Input: part model. Units: mm. Frame: model coordinates. A direction names the side the tool comes from. Round coordinates to 2 decimals unless told otherwise and drop trailing zeros. Write each loop counter-clockwise with the first axis right and the second up, starting at its lowest first coordinate (ties: lowest second). Pieces come first, ordered by that corner, then holes. Notation, with made-up numbers: (62, 26.25) -> (95, 26.25) arc R7 cw to (95, 35.25) -> close; hole circle Ø1 at (36, 61). An arc over 180 degrees is marked (long way). Use CSV: the item, a comma, the result in double quotes.
Autodesk Inventor part; units mm, degrees
ref_plane "Arbeitsebene1" through (-276.74, -145.36, 4.8625) normal (0, 0, 1) x (1, 0, 0)
ref_plane "YZ Plane" through (0, 0, 0) normal (1, 0, 0) x (0, 1, 0)
ref_plane "XZ Plane" through (0, 0, 0) normal (0, 1, 0) x (-1, 0, 0)
sketch "Skizze1" plane through (0, 0, 0) normal (0, 0, 1) x (1, 0, 0)
  circle A0 centre (-271.1, -102.4) radius 2.25
  circle A1 centre (-271, -139.7) radius 2.25
  circle A2 centre (-140.5, -84.3) radius 2.25
  circle A3 centre (-161.5, -132.1) radius 2.25
  circle A4 centre (-28.4, -139.7) radius 2.25
  circle A5 centre (-28.2, -86.4) radius 2.25
  circle A6 centre (-216.6, -72.6) radius 2.25
  point P0 (0, 0)
extrude "Extrusion1" add sketch "Skizze1" along normal blind 3 contours A0 | A1 | A2 | A3 | A4 | A5
sketch "Skizze2" plane through (-216.6, -72.6, 3) normal (0, 0, 1) x (1, 0, 0)
  line L0 (-57.14, 7.74) -> (190.86, 7.74)
  arc A0 (192.36, 6.24) -> (190.86, 7.74) centre (190.86, 6.24) ccw
  line L1 (192.36, 6.24) -> (192.36, -69.76)
  arc A1 (190.86, -71.26) -> (192.36, -69.76) centre (190.86, -69.76) ccw
  line L2 (190.86, -71.26) -> (-57.14, -71.26)
  arc A2 (-58.64, -69.76) -> (-57.14, -71.26) centre (-57.14, -69.76) ccw
  line L3 (-58.64, -69.76) -> (-58.64, 6.24)
  arc A3 (-57.14, 7.74) -> (-58.64, 6.24) centre (-57.14, 6.24) ccw
  point P0 (216.6, 72.6)
ref_plane "Arbeitsebene1" through (-276.74, -145.36, 4.8625) normal (0, 0, 1) x (1, 0, 0)
extrude "Extrusion2" add sketch "Skizze2" along normal up to surface (1.8625 mm away)
sketch "Skizze3" plane through (-273.74, -143.86, 4.8625) normal (0, 0, 1) x (1, 0, 0)
  line L0 (248, 80.5) -> (0, 80.5)
  arc A0 (0, 80.5) -> (-3, 77.5) centre (0, 77.5) ccw
  line L1 (-3, 77.5) -> (-3, 1.5)
  arc A1 (-3, 1.5) -> (0, -1.5) centre (0, 1.5) ccw
  line L2 (0, -1.5) -> (248, -1.5)
  arc A2 (248, -1.5) -> (251, 1.5) centre (248, 1.5) ccw
  line L3 (251, 1.5) -> (251, 77.5)
  arc A3 (251, 77.5) -> (248, 80.5) centre (248, 77.5) ccw
  point P0 (273.74, 143.86)
extrude "Extrusion3" add sketch "Skizze3" along normal blind 5
sketch "Skizze4" plane through (-273.74, -143.86, 9.8625) normal (0, 0, 1) x (1, 0, 0)
  circle A0 centre (245.54, 57.46) radius 2.25 construction
  circle A1 centre (245.34, 4.16) radius 2.25 construction
  circle A2 centre (133.24, 59.56) radius 1.2295
  circle A3 centre (133.24, 59.56) radius 1.2295
  circle A4 centre (112.24, 11.76) radius 1.6
  circle A5 centre (57.14, 71.26) radius 2.25
  circle A6 centre (2.64, 41.46) radius 1.2295
  circle A7 centre (2.74, 4.16) radius 1.2295
  circle A8 centre (2.64, 41.46) radius 2.85
  circle A9 centre (2.74, 4.16) radius 2.85
  circle A10 centre (57.14, 71.26) radius 2.85
  circle A11 centre (112.24, 11.76) radius 2.25
  circle A12 centre (112.24, 11.76) radius 2.85
  circle A13 centre (133.24, 59.56) radius 2.25
  circle A14 centre (133.24, 59.56) radius 2.85
  circle A15 centre (245.54, 57.46) radius 2.85
  circle A16 centre (245.34, 4.16) radius 2.85
  point P0 (273.74, 143.86)
  dimension "d6" = 5.7
  dimension "d7" = 5.7
  dimension "d8" = 5.7
  dimension "d9" = 5.7
  dimension "d10" = 5.7
  dimension "d11" = 5.7
  dimension "d12" = 5.7
extrude "Extrusion4" cut sketch "Skizze4" against normal blind 3.2 contours A2 | A4 | A6 | A7 | A8 | A9 | A11 | A12 | A13 | A14 | A15 | A16
sketch "Skizze5" plane through (-273.74, -143.86, 9.8625) normal (0, 0, 1) x (1, 0, 0)
  circle A0 centre (245.54, 57.46) radius 2.85
  circle A1 centre (245.34, 4.16) radius 2.85
  circle A2 centre (112.24, 11.76) radius 2.85
  circle A3 centre (133.24, 59.56) radius 2.85
  circle A4 centre (57.14, 71.26) radius 2.85
  circle A5 centre (2.64, 41.46) radius 2.85
  circle A6 centre (2.74, 4.16) radius 2.85
  point P0 (273.74, 143.86)
hole "Bohrung1" at (-271, -139.7, 9.8625) at (-271.1, -102.4, 9.8625) at (-161.5, -132.1, 9.8625) at (-140.5, -84.3, 9.8625) at (-28.2, -86.4, 9.8625) at (-28.4, -139.7, 9.8625) direction (0, 0, -1) diameter 3.2 depth 23.862
sketch "Skizze6" plane through (-273.74, -143.86, 9.8625) normal (0, 0, 1) x (1, 0, 0)
  circle A0 centre (245.54, 57.46) radius 2.85
  circle A1 centre (112.24, 11.76) radius 2.85
  circle A2 centre (2.74, 4.16) radius 2.85
  circle A3 centre (245.34, 4.16) radius 2.85
  circle A4 centre (133.24, 59.56) radius 2.85
  circle A5 centre (2.64, 41.46) radius 2.85
  arc A6 (0, 80.5) -> (-3, 77.5) centre (0, 77.5) ccw
  line L0 (-3, 77.5) -> (-3, 1.5)
  arc A7 (-3, 1.5) -> (0, -1.5) centre (0, 1.5) ccw
  line L1 (0, -1.5) -> (248, -1.5)
  arc A8 (248, -1.5) -> (251, 1.5) centre (248, 1.5) ccw
  line L2 (251, 1.5) -> (251, 77.5)
  arc A9 (251, 77.5) -> (248, 80.5) centre (248, 77.5) ccw
  line L3 (248, 80.5) -> (0, 80.5)
  point P0 (273.74, 143.86)
extrude "Extrusion5" add sketch "Skizze6" along normal blind 5
sketch "Skizze7" plane through (-22.74, -142.36, 4.8625) normal (1, 0, 0) x (0, 0, -1)
  line L0 (-10, 0) -> (-10, 76)
  line L1 (-10, 0) -> (-10, -3)
  line L2 (0, -3) -> (-10, -3)
  line L3 (0, 79) -> (-10, 79)
  line L4 (-10, 79) -> (-10, 76)
  line L5 (-10, 79) -> (-5.5, -3)
  point P0 (4.8625, 142.36)
  dimension "d27" = 4.5
extrude "Extrusion6" cut sketch "Skizze7" against normal through all
properties part number "Bottom"
Item 1: Section query B-B on y = -112. Return the cut outline in (x, z), plus the area to 3 significant figures.
Worked answers:
outline,"(-276.74, 4.86) -> (-275.24, 4.86) -> (-275.24, 3) -> (-24.24, 3) -> (-24.24, 4.86) -> (-22.74, 4.86) -> (-22.74, 12.19) -> (-276.74, 12.19) -> close"
area,"2,330 mm²"
Item 2: First-contact query: pin 1 Ø2.5 at (x, y) = (-28.4, -139.7) entering from -Z; pin 2 Ø4 at (x, y) = (-271.1, -102.4) entering from -Z; pin 3 Ø0.9 at (x, z) = (-119, 4) entering from -Y; pin 4 Ø0.6 at (y, z) = (-103, 3.5) entering from -X. Flat tips, straight axial feed; report the tip coordinate or a pass-through.
Worked answers:
pin 1,"passes through"
pin 2,"stops at z = 0"
pin 3,"stops at y = -143.86"
pin 4,"stops at x = -275.24"
Item 3: Section query A-A on x = -107. Return the cut outline in (y, z), plus the area to 3 significant figures.
Worked answers:
outline,"(-145.36, 4.86) -> (-143.86, 4.86) -> (-143.86, 3) -> (-64.86, 3) -> (-64.86, 4.86) -> (-63.36, 4.86) -> (-63.36, 14.86) -> (-145.36, 10.36) -> close"
area,"783 mm²"
Item 4: Pull-direction query (X, two-part tool) for faces 1 (the face through (-150.3, -64.7, 4.862)), 2 (the face through (-30.448, -86.499, 1.479)), 3 (the face through (-276.74, -104, 9)); classes: +X half, -X half, draft (parallel to the pull), parting line (faces both ways), or undercut.
Worked answers:
face 1,"draft"
face 2,"undercut"
face 3,"-X half"
Item 5: Set-up query: faces 4 (the face through (-273.248, -139.799, 1.479)), 5 (the face through (-162.12, -129.32, 8.92)), 6 (the face through (-273, -140, 0)). Return all of +Z, -Z, +X, -X, +Y, -Y with unobstructed straight access to the full face (end or side cutting, diameter ignored); none if empty.
Worked answers:
face 4,"-Z"
face 5,"+Z"
face 6,"-Z, +X, -X, +Y, -Y"
Item 6: Line query: line 1 (Y direction, x = -271, z = 7.75); line 2 (Y direction, x = -28.2, z = 10.25); line 3 (Y direction, x = -161.5, z = 9.8). Output: solid intervals per line, ascending.
Worked answers:
line 1,"y = -145.36 to -142.55, -136.85 to -105.25, -99.55 to -63.36"
line 2,"y = -145.36 to -142.54, -136.86 to -89.25, -83.55 to -63.36"
line 3,"y = -145.36 to -134.95, -129.25 to -63.36"
